Source: three-view drawing plus pictorial views. Frame: mm from the lowest corner of the part. A direction names the side the tool comes from. Round coordinates to 2 decimals unless told otherwise and drop trailing zeros. Order: outer loops, then holes, each group sorted by start corner. A loop starts at its lowest first (then second) coordinate and runs counter-clockwise, first axis right, second up. Notation, with made-up numbers: (8.5, -7.5) -> (56.5, -7.5) arc R17 ccw to (56.5, 6.5) -> close; hole circle Ø3 at (8, 66). An arc over 180 degrees is marked (long way). Answer as CSV lines item,"result". Start each with the question number.
1) Section query A-A, the plane z = 17. Output: boundary loops of the cut face in (x, y).
2) Access query for the marked faces 4 and 5. Directions: +Z, -Z, +X, -X, +Y, -Y. A direction counts if a zero-diameter tool reaches every point of the face in a straight line with its end or side. Return the directions, or none.
3) Section query B-B, the plane x = 14.75. Output: boundary loops of the cut face in (y, z).
4) Mould query, pull axis X, two halves, no side actions, for the marked faces 1, 2 and 3. Classes: +X half, -X half, draft (parallel to the pull), parting line (faces both ways), or undercut.
5) Section query C-C, the plane y = 3.25. State how many separate pieces and enclosed holes the cut face has, and give its area (3 significant figures).
6) First-contact query: P1, Ø4.5, axis at y = 10, z = 11.5, coming from the -X side; P2, Ø3, axis at x = 3, y = 4, coming from the -Z side; P3, Ø1.9, axis at x = 16, z = 4, coming from the -Y side; P4, Ø3, axis at x = 7.5, z = 28, coming from the -Y side. Flat tips, straight axial feed; report the tip coordinate or a pass-through.
7) Line query: L1, parallel to X at y = 7.75, z = 30; L2, parallel to X at y = 8.5, z = 4; L3, parallel to Z at x = 16, y = 4.25. Output: solid intervals per line, ascending.
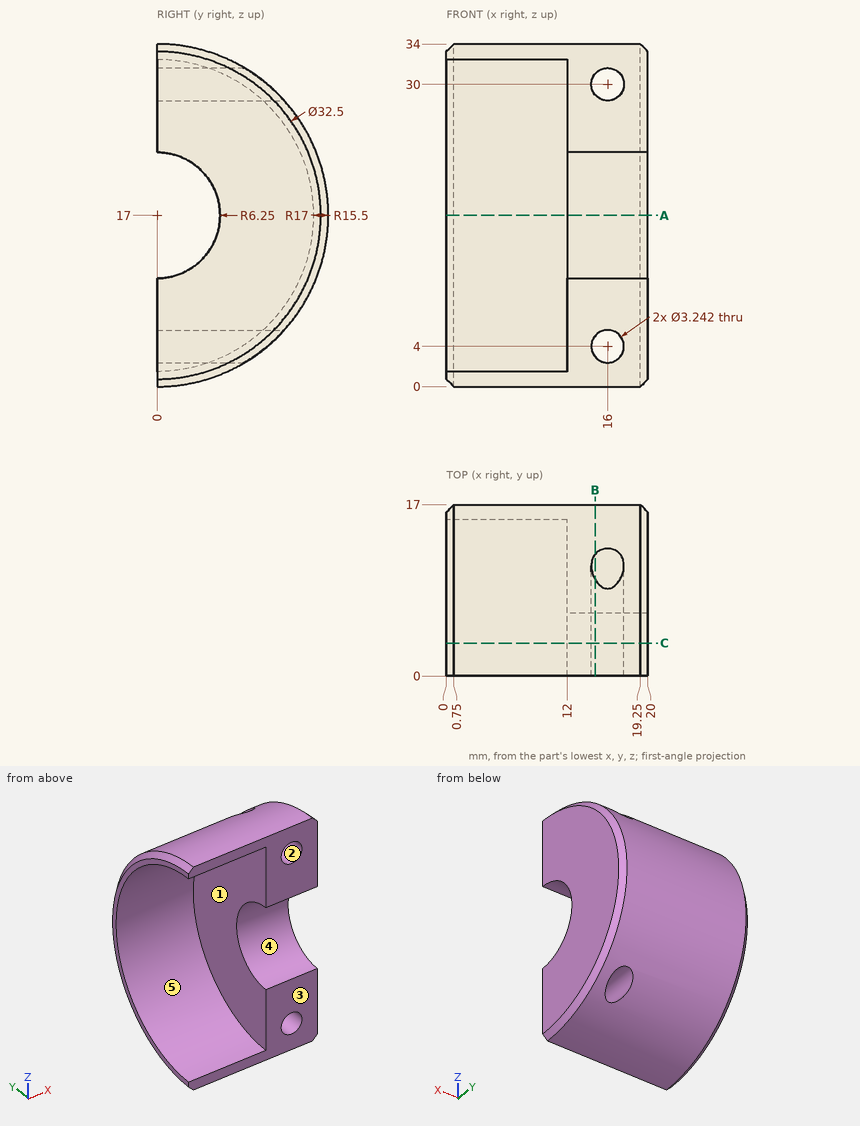
Findings:
1,outline,"(0, 15.5) -> (12, 15.5) -> (12, 6.25) -> (20, 6.25) -> (20, 16.25) -> (19.25, 17) -> (0.75, 17) -> (0, 16.25) -> close"
2,face 4,"+X, -X, -Y"
2,face 5,"-X, -Y"
3,outline,"(0, 0) arc R17 ccw to (9.6, 2.97) -> (0, 2.97) -> close; (0, 5.03) -> (12.07, 5.03) arc R17 ccw to (12.07, 28.97) -> (0, 28.97) -> (0, 23.25) arc R6.25 cw to (0, 10.75) -> close; (0, 31.03) -> (9.6, 31.03) arc R17 ccw to (0, 34) -> close"
4,face 1,"-X half"
4,face 2,"undercut"
4,face 3,"draft"
5,separate pieces,"2"
5,enclosed holes,"2"
5,area,"201 mm^2"
6,P1,"stops at x = 12"
6,P2,"stops at z = 0.18"
6,P3,"passes through"
6,P4,"stops at y = 9.17"
7,L1,"x = 12 to 14.38, 17.62 to 20"
7,L2,"x = 0 to 14.38, 17.62 to 20"
7,L3,"z = 0.54 to 2.38, 5.62 to 12.42, 21.58 to 28.38, 31.62 to 33.46"
